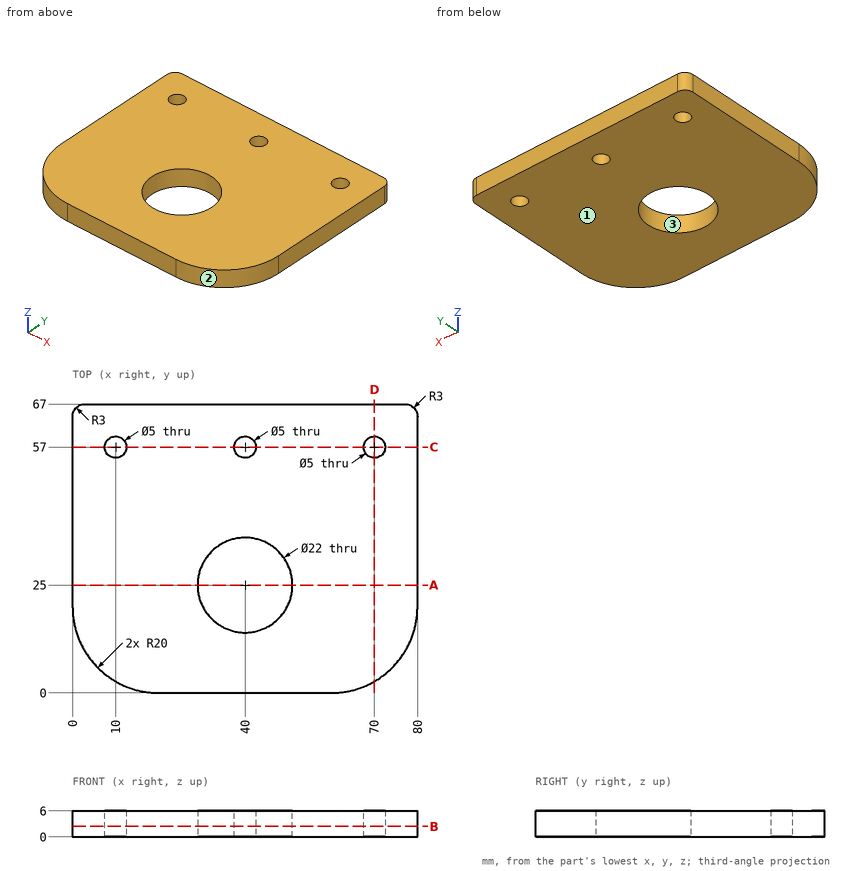
Part print with two shaded views. Sizes in mm from the minimum x, y, z corner. Round coordinates to 2 decimals unless told otherwise and drop trailing zeros. Loops run counter-clockwise (first coordinate to the right, second up) from the corner with the lowest first, then second, coordinate; pieces in that order, holes last. Notation, with made-up numbers: (19.25, -0.5) - (44.25, -0.5) arc R29 ccw to (44.25, 23.5) - close; hole circle Ø10 at (85, 42). An arc over 180 degrees is marked (long way). Put each result on its own line as item: value.
1. Wall check: line 1 (Y direction, x = 40, z = 4.35); line 2 (Y direction, x = 10, z = 4.75); line 3 (X direction, y = 23, z = 2.8). Give the ranges that are in metal, low to high.
Geometry check:
line 1: 0 to 14, 36 to 54.5, 59.5 to 67
line 2: 2.68 to 54.5, 59.5 to 67
line 3: 0 to 29.18, 50.82 to 80
2. Pin check, flat tips, straight feed: P1, Ø3, axis at y = 43.5, z = 1, coming from the -X side; P2, Ø3, axis at y = 12, z = 1.5, coming from the -X side; P3, Ø1, axis at y = 8.5, z = 3, coming from the -X side. Stop position of each tip, or through.
Geometry check:
P1: x = 0
P2: x = 1.09
P3: x = 3.3
3. Two-plate mould, pull along Y, no slides. Class the marked faces 1, 2 and 3: released by +Y, released by -Y, zero draft, split by the parting line, or undercut.
Geometry check:
face 1: zero draft
face 2: released by -Y
face 3: undercut
4. Slice it at D-D on x = 70. List the corners of the cut face in (y, z), and give its area (3 significant figures).
Geometry check:
outline: (2.68, 0) - (54.5, 0) - (54.5, 6) - (2.68, 6) - close; (59.5, 0) - (67, 0) - (67, 6) - (59.5, 6) - close
area: 356 mm²
5. Slice it at C-C on y = 57. List the corners of the cut face in (x, z), and give its area (3 significant figures).
Geometry check:
outline: (0, 0) - (7.5, 0) - (7.5, 6) - (0, 6) - close; (12.5, 0) - (37.5, 0) - (37.5, 6) - (12.5, 6) - close; (42.5, 0) - (67.5, 0) - (67.5, 6) - (42.5, 6) - close; (72.5, 0) - (80, 0) - (80, 6) - (72.5, 6) - close
area: 390 mm²
6. Slice it at B-B on z = 2.45. List the corners of the cut face in (x, y).
Geometry check:
outline: (0, 20) arc R20 ccw to (20, 0) - (60, 0) arc R20 ccw to (80, 20) - (80, 64) arc R3 ccw to (77, 67) - (3, 67) arc R3 ccw to (0, 64) - close; hole circle Ø5 at (10, 57); hole circle Ø22 at (40, 25); hole circle Ø5 at (40, 57); hole circle Ø5 at (70, 57)
7. Slice it at A-A on y = 25. List the corners of the cut face in (x, z), and give its area (3 significant figures).
Geometry check:
outline: (0, 0) - (29, 0) - (29, 6) - (0, 6) - close; (51, 0) - (80, 0) - (80, 6) - (51, 6) - close
area: 348 mm²
